from build123d import *

# Parameters (mm, degrees)
F4_DEPTH = 10.668


with BuildPart() as f2:
    # F0 (on Front) → F2 (revolve)
    with BuildSketch(Plane.XZ):
        Polygon((-45.128793, 24.239482), (-48.873104, 10.641724), (0, 10.641724), (0, 26.40724), (-10.838794, 26.40724), (-17.145, 13.597758), (-31.728104, 18.524483), (-34.881208, 31.333964), (-51.829137, 31.333964), align=None)
    revolve(axis=Axis((-26.604312, 0, 0), (1, 0, 0)))

    # F3 (on Right) → F4 (join)
    with BuildSketch(Plane.YZ):
        Polygon((34.092929, 0), (25.816033, 0), (24.436556, -10.050518), align=None)
    extrude(amount=-F4_DEPTH)


solid = f2.part
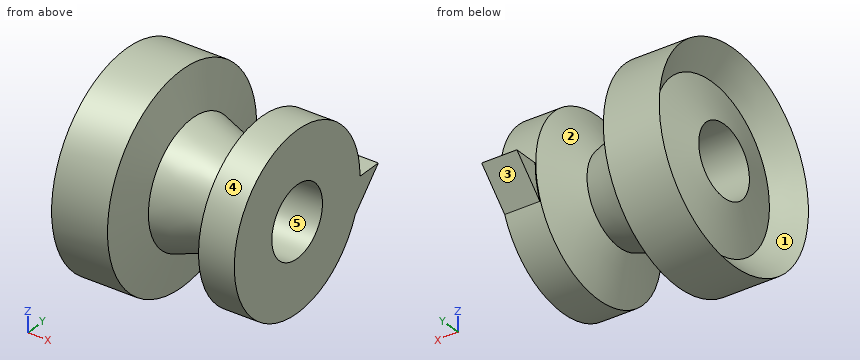
Source: CAD feature listing. Evaluate the final solid. Frame: model axes, mm. Face numbers are marked on the shaded views. A direction names the side the tool comes from. Give positions to 0.01 mm unless a question says otherwise; leave off trailing zeros. Write each loop counter-clockwise with the first axis right and the second up, starting at its lowest first coordinate (ties: lowest second). Pieces come first, ordered by that corner, then holes. Notation, with made-up numbers: M -29,56.25 L 0,56.25 A34 cw 0,91.25 Z; hole C 60.25,-24 d6. An arc over 180 degrees is marked long. Return JSON: item names as keys, results as strings. Group by question number.
1) First-contact query: pin 1 Ø12 at (x, y) = (-14, 12.5) entering from +Z; pin 2 Ø8 at (y, z) = (18.5, 6.5) entering from -X; pin 3 Ø2 at (x, z) = (-39.5, -18) entering from -Y; pin 4 Ø13 at (y, z) = (0, 0) entering from +X. Flat tips, straight axial feed; report the tip coordinate or a pass-through.
2) Cut plane A-A, the plane y = 0. Output: boundary loops of the cut face in (x, z) (3 decimals).
3) Ray query, L1, parallel to Z at x = -38.5, y = 0; L2, parallel to Z at x = -17.5, y = 0; L3, parallel to X at y = 13, z = 17.5. Return the intervals inside material, ascending.
4) Set-up query: the marked faces 1 and 2. Return all of +Z, -Z, +X, -X, +Y, -Y with unobstructed straight access to the full face (end or side cutting, diameter ignored); none if empty.
5) Draft query along Z for the marked faces 3, 4 and 5. Return one class per face: released by +Z, released by -Z, zero draft, split by the parting line, or undercut.
6) Cut plane B-B, the plane x = -27.5. Output: boundary loops of the cut face in (y, z), then the cut area to 3 significant figures.
Data:
{
 "1": {"pin 1": "stops at z = 25.35", "pin 2": "stops at x = -47.51", "pin 3": "stops at y = -26.32", "pin 4": "passes through"},
 "2": {"outline": "M -51.829,-31.334 L -34.881,-31.334 L -31.728,-18.524 L -17.145,-13.598 L -10.839,-26.407 L 0,-26.407 L 0,-10.642 L -48.873,-10.642 L -45.129,-24.239 Z; M -51.829,31.334 L -45.129,24.239 L -48.873,10.642 L 0,10.642 L 0,26.407 L -10.839,26.407 L -17.145,13.598 L -31.728,18.524 L -34.881,31.334 Z"},
 "3": {"L1": "z = -31.33 to -10.64, 10.64 to 31.33", "L2": "z = -13.72 to -10.64, 10.64 to 13.72", "L3": "x = -45.8 to -32.53, -13.11 to 0"},
 "4": {"face 1": "-X", "face 2": "none"},
 "5": {"face 3": "released by -Z", "face 4": "split by the parting line", "face 5": "undercut"},
 "6": {"outline": "C 0,0 d34.19; hole C 0,0 d21.28", "area": "562 mm²"}
}
